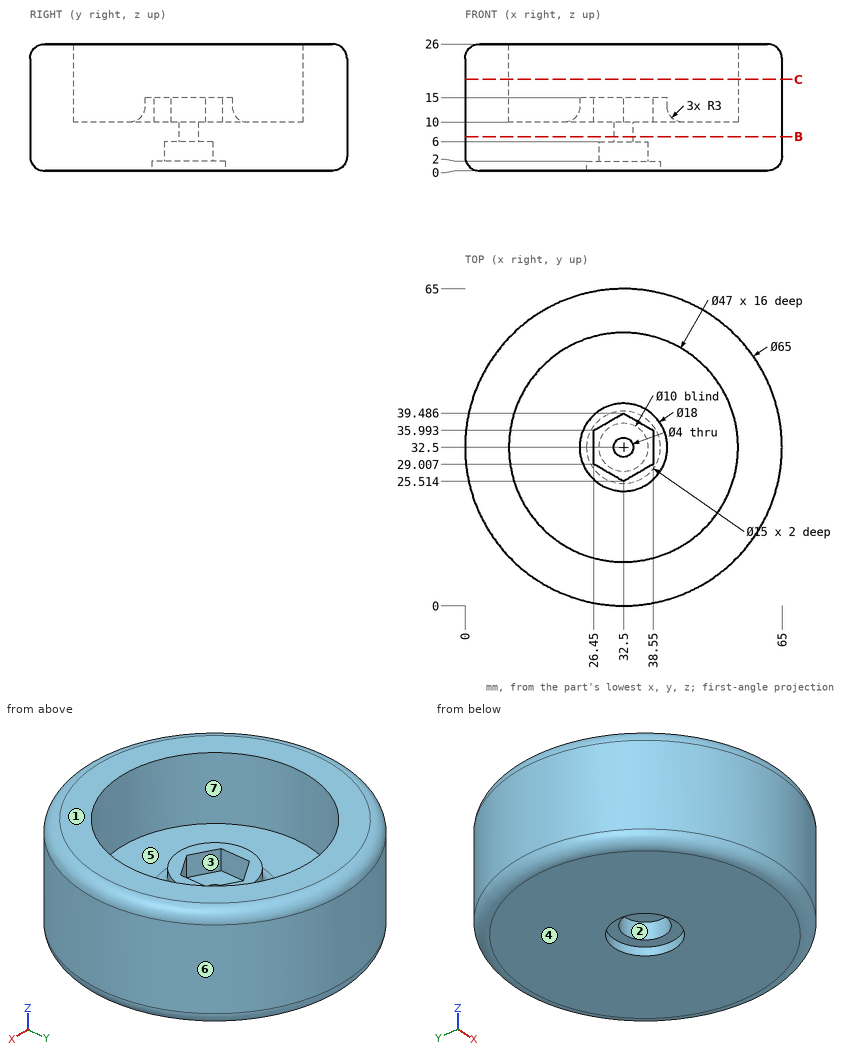
Geometry: see drawing. Coordinates: mm, zero at the bounding-box minimum. A direction names the side the tool comes from. Give positions to 0.01 mm unless a question says otherwise; leave off trailing zeros. Order: outer loops, then holes, each group sorted by start corner. A loop starts at its lowest first (then second) coordinate and runs counter-clockwise, first axis right, second up. Notation, with made-up numbers: (-6.75, 10.25) -> (13.25, 10.25) arc R24 ccw to (13.25, 41.25) -> close; hole circle Ø3 at (-2, -27.5). An arc over 180 degrees is marked (long way). Write each question's results on one line, items separated by ' | '.
1) Line query: line 1 along Y through (x, z) = (33, 19); line 2 along Y through (x, z) = (13, 12.75) (1 decimal); line 3 along Z through (x, y) = (30, 30). Output: solid intervals per line, ascending.
Geometry says:
line 1: y = 0 to 9.01, 55.99 to 65 | line 2: y = 6.5 to 19.4, 45.6 to 58.5 | line 3: z = 6 to 10
2) Cut plane B-B (z = 7). Output: boundary loops of the cut face in (x, y), and give its area (3 significant figures).
Geometry says:
outline: circle Ø65 at (32.5, 32.5); hole circle Ø4 at (32.5, 32.5) | area: 3,310 mm²
3) Draft query along X for the marked faces 4, 5, 6 and 7. Return one class per face: released by +X, released by -X, zero draft, split by the parting line, or undercut.
Geometry says:
face 4: zero draft | face 5: undercut | face 6: split by the parting line | face 7: undercut
4) Set-up query: the marked faces 1, 2 and 3. Return all of +Z, -Z, +X, -X, +Y, -Y with unobstructed straight access to the full face (end or side cutting, diameter ignored); none if empty.
Geometry says:
face 1: +Z, +X, -X, +Y, -Y | face 2: -Z | face 3: +Z
5) Cut plane C-C (z = 18.75). Output: boundary loops of the cut face in (x, y), and give its area (3 significant figures).
Geometry says:
outline: circle Ø65 at (32.5, 32.5); hole circle Ø47 at (32.5, 32.5) | area: 1,580 mm²
6) First-contact query: pin 1 Ø6 at (y, z) = (26, 3) entering from +X; pin 2 Ø6.5 at (x, y) = (32.5, 32.5) entering from -Z; pin 3 Ø10 at (x, y) = (36.5, 32) entering from +Z; pin 4 Ø1.5 at (y, z) = (33, 11.5) entering from +X. Flat tips, straight axial feed; report the tip coordinate or a pass-through.
Geometry says:
pin 1: stops at x = 64.81 | pin 2: stops at z = 6 | pin 3: stops at z = 15 | pin 4: stops at x = 65
